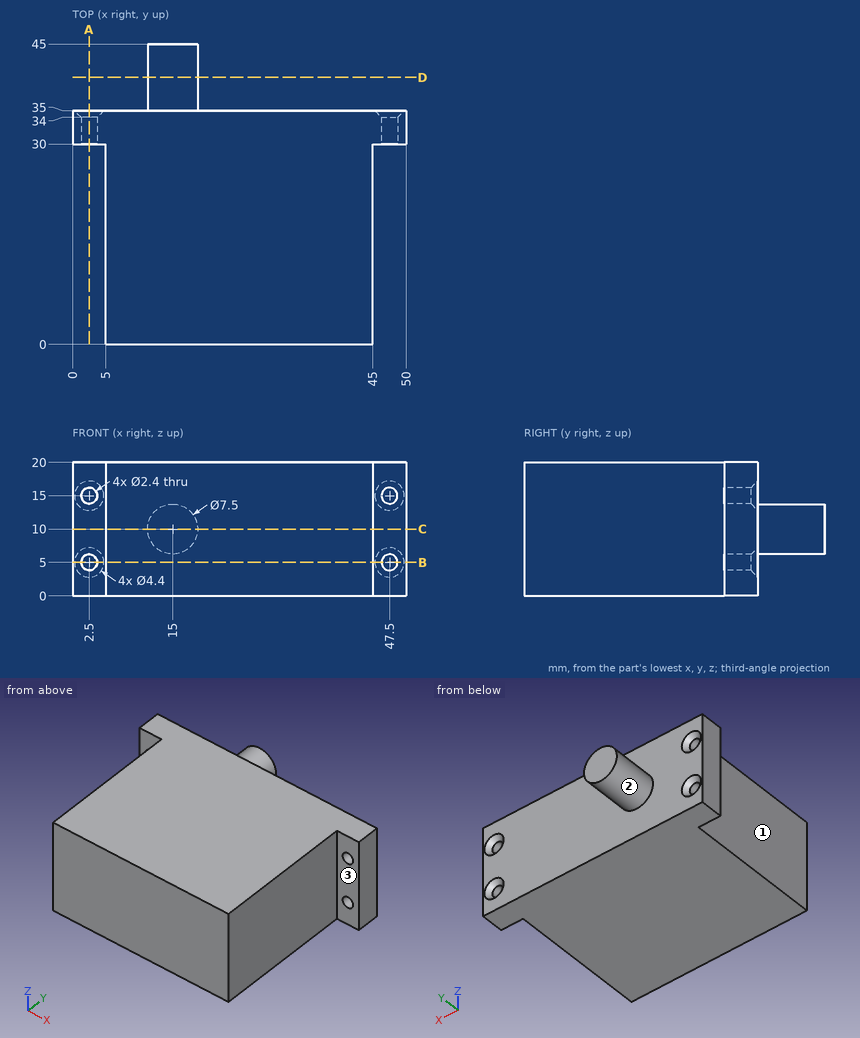
Can you work these out from the drawing? Everything is in mm from the part's minimum corner. A direction names the side the tool comes from. Give positions to 0.01 mm unless a question says otherwise; leave off trailing zeros. Loops run counter-clockwise (first coordinate to the right, second up) from the corner with the lowest first, then second, coordinate; pieces in that order, holes last. Notation, with made-up numbers: (43.5, 41) - (53.5, 41) arc R16 ccw to (53.5, 69) - close; hole circle Ø3 at (-18, 52.25). An arc over 180 degrees is marked (long way). Use one line per item in the form item = value.
1. I want a section at A-A (x = 2.5). Please give me the cut outline in (y, z), and give its area (3 significant figures).
Response values:
outline = (30, 0) - (35, 0) - (35, 2.8) - (34, 3.8) - (30, 3.8) - close; (30, 6.2) - (34, 6.2) - (35, 7.2) - (35, 12.8) - (34, 13.8) - (30, 13.8) - close; (30, 16.2) - (34, 16.2) - (35, 17.2) - (35, 20) - (30, 20) - close
area = 74.0 mm²
2. I want a section at C-C (z = 10). Please give me the cut outline in (x, y).
Response values:
outline = (0, 30) - (5, 30) - (5, 0) - (45, 0) - (45, 30) - (50, 30) - (50, 35) - (18.75, 35) - (18.75, 45) - (11.25, 45) - (11.25, 35) - (0, 35) - close
3. On a 3-axis mill with a long thin cutter (end or side, diameter ignored), from which of +Z, -Z, +X, -X, +Y, -Y can I reach the whole of each face in a straight line? I mean the marked faces 1, 2 and 3. Say none if no direction works.
Response values:
face_1 = +Z, -Z, -X, -Y
face_2 = +Y
face_3 = +Z, -Z, +X, -Y
4. I need wall thicknesses on probe 1 along Z at (x, y) = (2.5, 31.3); probe 2 along Y at (x, z) = (20.5, 6); probe 3 along X at (y, z) = (19.5, 2.25). Which ranges of each line are inside material? Lowest first, please.
Response values:
probe_1 = 0 to 3.8, 6.2 to 13.8, 16.2 to 20
probe_2 = 0 to 35
probe_3 = 5 to 45
5. I'm going to push flat-ended pins straight in: pin 1 Ø3 at (x, z) = (42.5, 16.5) entering from -Y; pin 2 Ø2 at (y, z) = (25, 5.5) entering from +X; pin 3 Ø1 at (y, z) = (21, 9) entering from -X; pin 4 Ø1.5 at (x, z) = (3, 11) entering from -Y. Where does each tip first touch, or does it pass through?
Response values:
pin_1 = 0
pin_2 = 45
pin_3 = 5
pin_4 = 30
6. I want a section at D-D (y = 40). Please give me the cut outline in (x, z).
Response values:
outline = circle Ø7.5 at (15, 10)
7. I want a section at B-B (z = 5). Please give me the cut outline in (x, y), and give its area (3 significant figures).
Response values:
outline = (0, 30) - (1.3, 30) - (1.3, 34) - (0.3, 35) - (0, 35) - close; (3.7, 30) - (5, 30) - (5, 0) - (45, 0) - (45, 30) - (46.3, 30) - (46.3, 34) - (45.3, 35) - (4.7, 35) - (3.7, 34) - close; (48.7, 30) - (50, 30) - (50, 35) - (49.7, 35) - (48.7, 34) - close
area = 1,420 mm²
